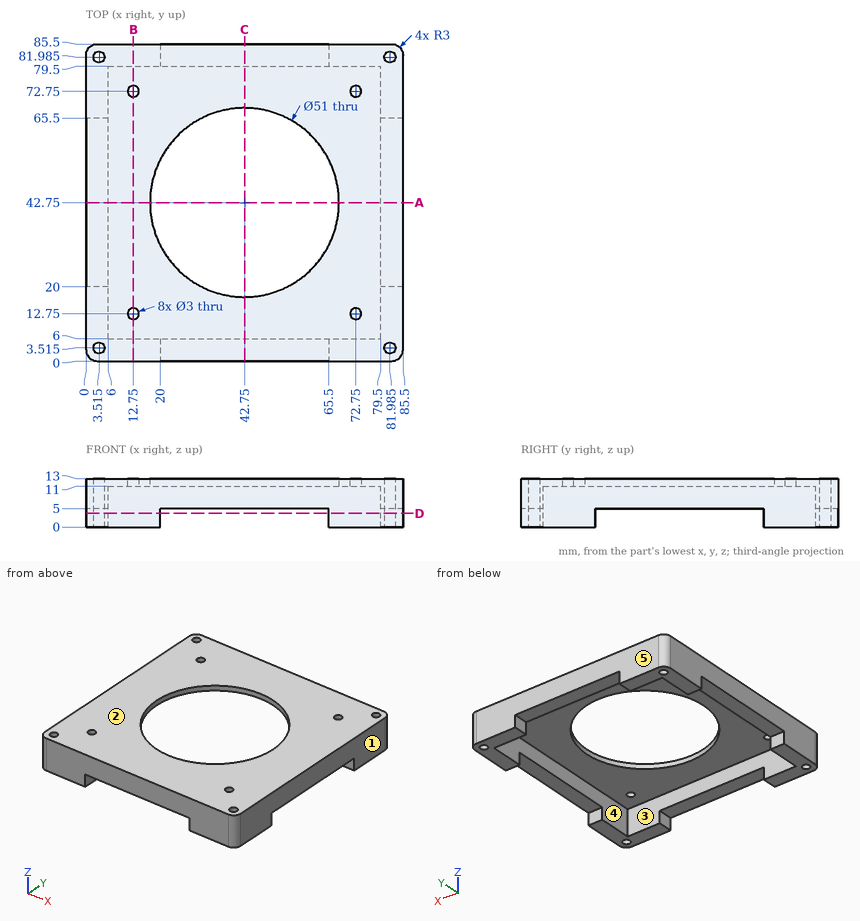
Input: dimensioned drawing with shaded views. Units: mm. Origin: part minimum x, y, z. A direction names the side the tool comes from. Give positions to 0.01 mm unless a question says otherwise; leave off trailing zeros. Write each loop counter-clockwise with the first axis right and the second up, starting at its lowest first coordinate (ties: lowest second). Pieces come first, ordered by that corner, then holes. Notation, with made-up numbers: M 4.5,-38 L 27.5,-38 A29 cw 27.5,0 Z; hole C 53,-12 d2. An arc over 180 degrees is marked long. Return JSON: item names as keys, results as strings. Group by question number.
1) Pull-direction query (X, two-part tool) for the marked faces 1, 2 and 3; classes: pulls with the +X half, pulls with the -X half, needs draft (parallel to the pull), parting line crosses it, or undercut.
2) Cut plane B-B, the plane x = 12.75. Output: boundary loops of the cut face in (y, z).
3) Cut plane A-A, the plane y = 42.75. Output: boundary loops of the cut face in (x, z).
4) Material intervals for line 1 along X through (y, z) = (72.75, 11.5); line 2 along Y through (x, z) = (16.5, 4.5), sorted ascending. Write a range as [from, to].
5) Cut plane D-D, the plane z = 3.75. Give the number of separate pieces and of enclosed holes in the cut face, plus the area to 3 significant figures.
6) Set-up query: the marked faces 4 and 5. Return all of +Z, -Z, +X, -X, +Y, -Y with unobstructed straight access to the full face (end or side cutting, diameter ignored); none if empty.
7) Pin query (flat end, axial travel): P1, Ø5.5, axis at y = 3.5, z = 3.5, coming from the -X side; P2, Ø2.5, axis at x = 3.51, y = 81.99, coming from the +Z side; P3, Ø1.8, axis at x = 4.5, y = 53, coming from the -Z side. Return the tip coordinate at first contact, or that it passes through.
Recorded:
{
 "1": {"face 1": "pulls with the +X half", "face 2": "needs draft", "face 3": "undercut"},
 "2": {"outline": "M 0,0 L 6,0 L 6,11 L 11.25,11 L 11.25,13 L 0,13 Z; M 14.25,11 L 71.25,11 L 71.25,13 L 14.25,13 Z; M 74.25,11 L 79.5,11 L 79.5,0 L 85.5,0 L 85.5,13 L 74.25,13 Z"},
 "3": {"outline": "M 0,5 L 6,5 L 6,11 L 17.25,11 L 17.25,13 L 0,13 Z; M 68.25,11 L 79.5,11 L 79.5,5 L 85.5,5 L 85.5,13 L 68.25,13 Z"},
 "4": {"line 1": "x = [0, 11.25], [14.25, 71.25], [74.25, 85.5]", "line 2": "y = [0, 6], [79.5, 85.5]"},
 "5": {"separate pieces": "4", "enclosed holes": "4", "area": "780 mm²"},
 "6": {"face 4": "-Z", "face 5": "+Z, -Z, +X, -X, +Y"},
 "7": {"P1": "stops at x = 0", "P2": "passes through", "P3": "stops at z = 5"}
}
